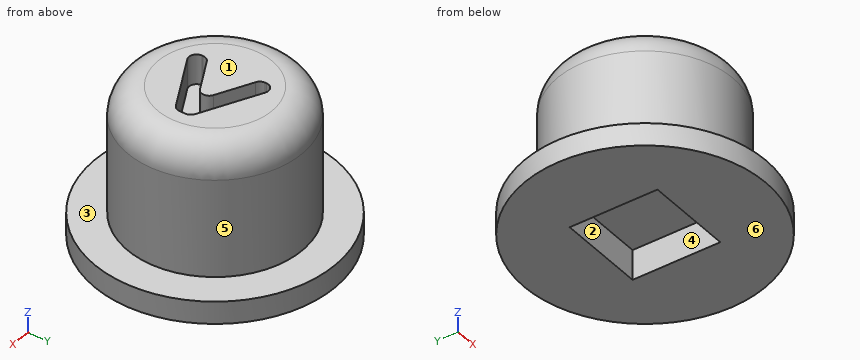
from build123d import *

# Parameters (mm, degrees)
SZKIC1_R                    = 4
DODANIE_WYCI_GNI_CIE1_DEPTH = 0.75
SZKIC2_R                    = 2.9
DODANIE_WYCI_GNI_CIE2_DEPTH = 4.25
SZKIC3_W                    = 2.5
SZKIC3_H                    = 2.5
WYTNIJ_WYCI_GNI_CIE1_DEPTH  = 1
ZAOKR_GLENIE2_R             = 1
SZKIC4_W                    = 2.9
SZKIC4_H                    = 2.9
WYTNIJ_WYCI_GNI_CIE2_DEPTH  = 1
WYTNIJ_WYCI_GNI_CIE3_DEPTH  = 1
ZAOKR_GLENIE3_R             = 0.25


with BuildPart() as part:
    # Szkic1 → Dodanie-wyciągnięcie1 (new body)
    with BuildSketch(Plane.XY):
        Circle(SZKIC1_R)
    extrude(amount=DODANIE_WYCI_GNI_CIE1_DEPTH)

    # Szkic2 → Dodanie-wyciągnięcie2 (add)
    with BuildSketch(Plane.XY.offset(0.75)):
        Circle(SZKIC2_R)
    extrude(amount=DODANIE_WYCI_GNI_CIE2_DEPTH)

    # Szkic3 → Wytnij-wyciągnięcie1 (cut)
    with BuildSketch(Plane(origin=(0, 0, 0), x_dir=(-1, 0, 0), z_dir=(0, 0, -1))):
        Rectangle(SZKIC3_W, SZKIC3_H)
    extrude(amount=-WYTNIJ_WYCI_GNI_CIE1_DEPTH, mode=Mode.SUBTRACT)

    # Zaokrąglenie2
    zaokr_glenie2_edges = [part.edges().sort_by_distance(p)[0] for p in [
        (-2.9, 0, 5),
    ]]
    fillet(zaokr_glenie2_edges, radius=ZAOKR_GLENIE2_R)

    # Szkic4 → Wytnij-wyciągnięcie2 (cut)
    with BuildSketch(Plane(origin=(0, 0, 0), x_dir=(-1, 0, 0), z_dir=(0, 0, -1))):
        Rectangle(SZKIC4_W, SZKIC4_H)
    extrude(amount=-WYTNIJ_WYCI_GNI_CIE2_DEPTH, mode=Mode.SUBTRACT)

    # Szkic5 → Wytnij-wyciągnięcie3 (cut)
    with BuildSketch(Plane.XY.offset(5)):
        Polygon((-0.902184432, 0.860277554), (-0.902184432, 1.46043781), (1.476020697, 0.234175791), (1.476020697, -0.263620684), (-0.902184432, -1.489181581), (-0.902184432, -0.889722446), (0.795231434, -0.014722446), align=None)
    extrude(amount=-WYTNIJ_WYCI_GNI_CIE3_DEPTH, mode=Mode.SUBTRACT)

    # Zaokrąglenie3
    zaokr_glenie3_edges = [part.edges().sort_by_distance(p)[0] for p in [
        (0.795231434, -0.014722446, 4.5),
        (-0.902184432, 0.860277554, 4.5),
        (-0.902184432, 1.46043781, 4.5),
        (1.476020697, 0.234175791, 4.5),
        (1.476020697, -0.263620684, 4.5),
        (-0.902184432, -1.489181581, 4.5),
        (-0.902184432, -0.889722446, 4.5),
    ]]
    fillet(zaokr_glenie3_edges, radius=ZAOKR_GLENIE3_R)


solid = part.part
Source: CAD feature listing. Evaluate the final solid. Frame: model axes, mm. Face numbers are marked on the shaded views. A direction names the side the tool comes from. Round coordinates to 2 decimals unless told otherwise and drop trailing zeros. Loops run counter-clockwise (first coordinate to the right, second up) from the corner with the lowest first, then second, coordinate; pieces in that order, holes last. Notation, with made-up numbers: (81.25, 38.5) - (96.25, 38.5) arc R17 cw to (96.25, 44.5) - close; hole circle Ø6 at (-35.75, 62). An arc over 180 degrees is marked (long way). Write item = value, one per line. Start each with the question number.
(1) Ray query, line 1 along Z through (x, y) = (-1.75, 3.5); line 2 along Z through (x, y) = (1, -1); line 3 along X through (y, z) = (-0.75, 4.2). Return the intervals inside material, ascending. Write a range as from..to.
(2) Pin query (flat end, axial travel): pin 1 (3 mm diameter, centred on y = -2, z = 2.5, fed in from -X); pin 2 (0.5 mm diameter, centred on y = 0.5, z = 0.5, fed in from +X); pin 3 (1 mm diameter, centred on x = 3, z = 3.5, fed in from -Y). Return the tip coordinate at first contact, or that it passes through.
(3) Section query B-B, the plane z = 2.4. Output: boundary loops of the cut face in (x, y), plus the area to 3 significant figures.
(4) Section query A-A, the plane x = 0. Output: boundary loops of the cut face in (y, z).
(5) Set-up query: the marked faces 1, 2 and 3. Return all of +Z, -Z, +X, -X, +Y, -Y with unobstructed straight access to the full face (end or side cutting, diameter ignored); none if empty.
(6) Section query C-C, the plane y = 3. Output: boundary loops of the cut face in (x, z).
(7) Pull-direction query (X, two-part tool) for the marked faces 4, 5 and 6; classes: +X half, -X half, draft (parallel to the pull), parting line (faces both ways), or undercut.
Conclusion:
q1.line_1 = 0..0.75
q1.line_2 = 1..5
q1.line_3 = -2.78..-0.63, 0.53..2.78
q2.pin_1 = -2.86
q2.pin_2 = 3.99
q2.pin_3 = -1.47
q3.outline = circle Ø5.8 at (0, 0)
q3.area = 26.4 mm2
q4.outline = (-4, 0) - (-1.45, 0) - (-1.45, 1) - (1.45, 1) - (1.45, 0) - (4, 0) - (4, 0.75) - (2.9, 0.75) - (2.9, 4) arc R1 ccw to (1.9, 5) - (1, 5) - (1, 4) - (0.4, 4) - (0.4, 5) - (-0.42, 5) - (-0.42, 4) - (-1.02, 4) - (-1.02, 5) - (-1.9, 5) arc R1 ccw to (-2.9, 4) - (-2.9, 0.75) - (-4, 0.75) - close
q5.face_1 = +Z, +X, -X, +Y, -Y
q5.face_2 = -Z
q5.face_3 = +Z
q6.outline = (-2.65, 0) - (2.65, 0) - (2.65, 0.75) - (-2.65, 0.75) - close
q7.face_4 = undercut
q7.face_5 = parting line
q7.face_6 = draft
